```python
from build123d import *

# Parameters (mm, degrees)
SKETCH_R           = 6.35
PAD_DEPTH          = 14.5
SKETCH001_R        = 1.45
POCKET_DEPTH       = 4.590236
SKETCH002_R        = 15.875
PAD001_DEPTH       = 2
SKETCH003_R        = 1.75
POCKET001_DEPTH    = 5
POLARPATTERN_COUNT = 4


with BuildPart() as part:
    # Sketch → Pad (new body)
    with BuildSketch(Plane.XY):
        Circle(SKETCH_R)
        with BuildLine():
            ThreePointArc((-1.651, 1.759764), (0, -2.413), (1.651, 1.759764))
            Line((-1.651, 1.759764), (1.651, 1.759764))
        make_face(mode=Mode.SUBTRACT)
    extrude(amount=PAD_DEPTH)

    # Sketch001 (on DatumPlane) → Pocket (cut)
    with BuildSketch(Plane.XZ.offset(-1.759764)):
        with Locations((0, 6.5)):
            Circle(SKETCH001_R)
    extrude(amount=-POCKET_DEPTH, mode=Mode.SUBTRACT)

    # Sketch002 (on Face3 of Pocket) → Pad001 (join)
    with BuildSketch(Plane.XY.offset(14.5)):
        Circle(SKETCH002_R)
    extrude(amount=PAD001_DEPTH)

    # Sketch003 (on Face3 of Pad001) → Pocket001 (cut)
    with BuildSketch(Plane.XY.offset(16.5)):
        with Locations((0, 10.795)):
            Circle(SKETCH003_R)
    pocket001 = extrude(amount=-POCKET001_DEPTH, mode=Mode.SUBTRACT)

    # PolarPattern: Pocket001 ×4 about axis
    polarpattern_axis = Axis((0, 0, 16.5), (0, 0, 1))
    for i in range(1, POLARPATTERN_COUNT):
        add(pocket001.rotate(polarpattern_axis, i * 360 / POLARPATTERN_COUNT), mode=Mode.SUBTRACT)


solid = part.part
```
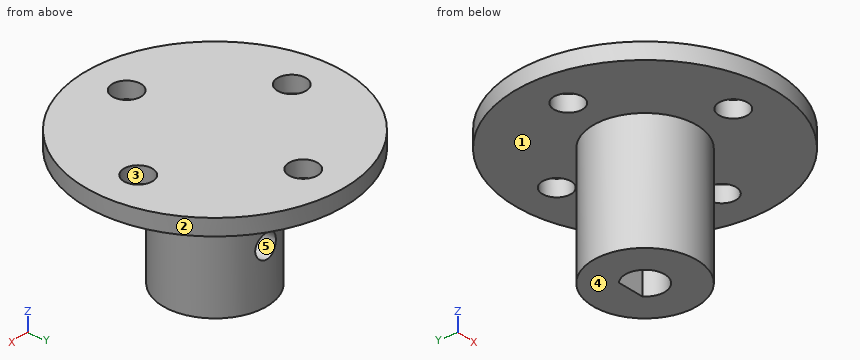
The model under review builds one solid part; all positions refer to its coordinate system, in mm. Face numbers are marked on the shaded views. A direction names the side the tool comes from. Coordinates: 2 decimals unless noted, no trailing zeros. Write each loop counter-clockwise with the first axis right and the second up, starting at its lowest first coordinate (ties: lowest second). Pieces come first, ordered by that corner, then holes. Notation, with made-up numbers: (15.5, 58.25) -> (42.5, 58.25) arc R29 cw to (42.5, 91.25) -> close; hole circle Ø9 at (85.5, 34.25). An arc over 180 degrees is marked (long way). One line per item, written item: value. Start each with the question number.
Q1. Clearance check with flat-ended pins moving along their axes: P1, Ø2, axis at y = -9, z = 8.5, coming from the +X side; P2, Ø1.5, axis at y = 4, z = 5, coming from the -X side; P3, Ø5.5, axis at x = 0, y = -10.795, coming from the -Z side; P4, Ø5, axis at x = -5, z = 10, coming from the -Y side. State where each tip first meets the part, or that it passes through.
Q2. Add section D-D, the plane z = 10. Give the boundary of the cut face in (x, y).
Q3. For the marked faces 1 and 2, list the 3-axis set-ups (+Z, -Z, +X, -X, +Y, -Y) from which the entire face can be reached by the end or side of a thin tool; tool diameter is ignored.
Q4. To check wall thickness, follow probe 1 along Z at (x, y) = (0, 2.75); probe 2 along Z at (x, y) = (10, 5); probe 3 along X at (y, z) = (2, 7). State the ranges of each line that lie inside material, in increasing order.
Q5. Add section B-B, the plane y = 0. Give the boundary of the cut face in (x, z) (3 decimals).
Q6. Add section A-A, the plane x = 0. Give the boundary of the cut face in (y, z) (3 decimals), then the cut area to 3 significant figures.
Q7. The part is to be moulded in two halves that separate along Z. For the marked faces 3, 4 and 5, say which applies: +Z half, -Z half, draft (parallel to the pull), parting line (faces both ways), or undercut.
Q8. Add section C-C, the plane y = 4. Give the boundary of the cut face in (x, z).
Response:
1. P1: through
1. P2: x = -5.46
1. P3: z = 14.5
1. P4: y = -5.84
2. outline: circle Ø12.7 at (0, 0); hole (-1.65, 1.76) arc R2.41 ccw (long way) to (1.65, 1.76) -> close
3. face 1: -Z
3. face 2: +Z, -Z
4. probe 1: 0 to 5.05, 7.95 to 16.5
4. probe 2: 14.5 to 16.5
4. probe 3: -6.03 to -1.36, 1.36 to 6.03
5. outline: (-15.875, 14.5) -> (-12.545, 14.5) -> (-12.545, 16.5) -> (-15.875, 16.5) -> close; (-9.045, 14.5) -> (-6.35, 14.5) -> (-6.35, 0) -> (-2.413, 0) -> (-2.413, 14.5) -> (2.413, 14.5) -> (2.413, 0) -> (6.35, 0) -> (6.35, 14.5) -> (9.045, 14.5) -> (9.045, 16.5) -> (-9.045, 16.5) -> close; (12.545, 14.5) -> (15.875, 14.5) -> (15.875, 16.5) -> (12.545, 16.5) -> close
6. outline: (-15.875, 14.5) -> (-12.545, 14.5) -> (-12.545, 16.5) -> (-15.875, 16.5) -> close; (-9.045, 14.5) -> (-6.35, 14.5) -> (-6.35, 0) -> (-2.413, 0) -> (-2.413, 14.5) -> (1.76, 14.5) -> (1.76, 7.95) -> (6.35, 7.95) -> (6.35, 14.5) -> (9.045, 14.5) -> (9.045, 16.5) -> (-9.045, 16.5) -> close; (1.76, 0) -> (6.35, 0) -> (6.35, 5.05) -> (1.76, 5.05) -> close; (12.545, 14.5) -> (15.875, 14.5) -> (15.875, 16.5) -> (12.545, 16.5) -> close
6. area: 160 mm²
7. face 3: draft
7. face 4: -Z half
7. face 5: undercut
8. outline: (-15.36, 14.5) -> (-4.93, 14.5) -> (-4.93, 0) -> (4.93, 0) -> (4.93, 14.5) -> (15.36, 14.5) -> (15.36, 16.5) -> (-15.36, 16.5) -> close; hole circle Ø2.9 at (0, 6.5)
